from build123d import *

# Parameters (mm, degrees)
F0_R     = 8.575
F1_DEPTH = 26.5
F3_DEPTH = 26.5


with BuildPart() as f1:
    # F0 (on Top) → F1 (new body)
    with BuildSketch(Plane.XY):
        Circle(F0_R)
    extrude(amount=F1_DEPTH)

    # F2 (on face) → F3 (cut)
    with BuildSketch(Plane(origin=(0, 0, 0), x_dir=(1, 0, 0), z_dir=(0, 0, -1))):
        Polygon((4.9857674621, 0.3769917955), (2.3840555737, 1.6277629909), (2.6017118884, -1.2507711954), align=None)
        Polygon((2.819368203, -4.1293053818), (2.6017118884, -1.2507711954), (0.2176563146, -2.8785341864), align=None)
        Polygon((0.2176563146, -2.8785341864), (-2.3840555737, -1.6277629909), (-2.1663992591, -4.5062971773), align=None)
        Polygon((-2.3840555737, -1.6277629909), (-2.6017118884, 1.2507711954), (-4.9857674621, -0.3769917955), align=None)
        Polygon((2.3840555737, 1.6277629909), (-0.2176563146, 2.8785341864), (-2.6017118884, 1.2507711954), (-2.3840555737, -1.6277629909), (0.2176563146, -2.8785341864), (2.6017118884, -1.2507711954), align=None)
        Polygon((2.1663992591, 4.5062971773), (-0.2176563146, 2.8785341864), (2.3840555737, 1.6277629909), align=None)
        Polygon((-0.2176563146, 2.8785341864), (-2.819368203, 4.1293053818), (-2.6017118884, 1.2507711954), align=None)
    extrude(amount=-F3_DEPTH, mode=Mode.SUBTRACT)


solid = f1.part
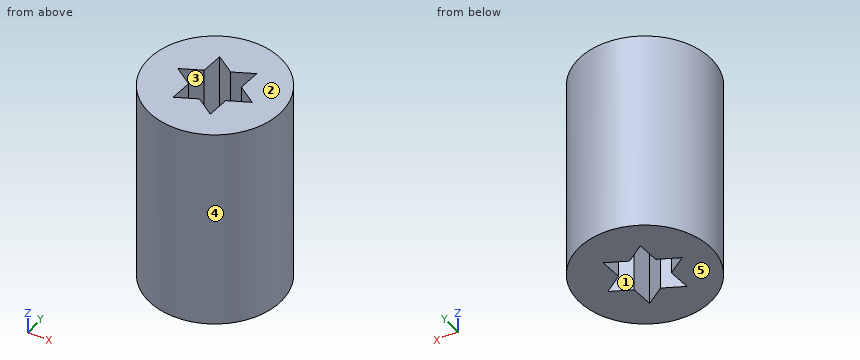
Design review of the part built by this model. Coordinates are the model's own, in mm. Face numbers are marked on the shaded views. A direction names the side the tool comes from. Round coordinates to 2 decimals unless told otherwise and drop trailing zeros. Write each loop counter-clockwise with the first axis right and the second up, starting at its lowest first coordinate (ties: lowest second). Pieces come first, ordered by that corner, then holes. Notation, with made-up numbers: (34.5, -9) - (82.5, -9) arc R14 ccw to (82.5, 7) - close; hole circle Ø6 at (60.5, 45). An arc over 180 degrees is marked (long way). Return JSON: item names as keys, results as strings. Group by question number.
Item 1: Machinability: for the marked faces 1 and 2, which of the approach directions +Z, -Z, +X, -X, +Y, -Y give a long, thin tool a straight path to every point of the face, cutting with its end or side? Answer none if there is none.
Item 2: The part is to be moulded in two halves that separate along Y. For the marked faces 3, 4 and 5, say which applies: pulls with the +Y half, pulls with the -Y half, needs draft (parallel to the pull), parting line crosses it, or undercut.
Item 3: We need section B-B on y = 0. Write out the cut boundary in (x, z) (3 decimals).
Item 4: We need section D-D on y = -5.75. Write out the cut boundary in (x, z), and give its area (3 significant figures).
Item 5: We need section A-A on z = 24.75. Write out the cut boundary in (x, y) (3 decimals), and give its area (3 significant figures).
Item 6: For probe 1 along X at (y, z) = (0.75, 2); probe 2 along X at (y, z) = (2, 13.75); probe 3 along Y at (x, z) = (3.5, 9), list the stretches that pass through material, from the lowest coordinate up. Write a range as [from, to].
Item 7: Insertion check: P1, Ø1, axis at x = 2.5, y = 0.5, coming from the -Z side; P2, Ø4, axis at y = -6.5, z = 13.5, coming from the -X side; P3, Ø2, axis at y = -3.5, z = 11, coming from the -X side; P4, Ø5, axis at y = -6, z = 8.5, coming from the -X side. Each pin has a flat end and moves straight along its axis. Give the tip position at first contact, or say it passes through.
Item 8: We need section C-C on y = 2. Write out the cut boundary in (x, z).
Model answer:
{
 "1": {"face 1": "+Z, -Z", "face 2": "+Z, +X, -X, +Y, -Y"},
 "2": {"face 3": "undercut", "face 4": "parting line crosses it", "face 5": "needs draft"},
 "3": {"outline": "(-8.575, 0) - (-4.434, 0) - (-4.434, 26.5) - (-8.575, 26.5) - close; (4.434, 0) - (8.575, 0) - (8.575, 26.5) - (4.434, 26.5) - close"},
 "4": {"outline": "(-6.36, 0) - (6.36, 0) - (6.36, 26.5) - (-6.36, 26.5) - close", "area": "337 mm²"},
 "5": {"outline": "circle Ø17.15 at (0, 0); hole (-4.986, 0.377) - (-2.602, -1.251) - (-2.819, -4.129) - (-0.218, -2.879) - (2.166, -4.506) - (2.384, -1.628) - (4.986, -0.377) - (2.602, 1.251) - (2.819, 4.129) - (0.218, 2.879) - (-2.166, 4.506) - (-2.384, 1.628) - close", "area": "188 mm²"},
 "6": {"probe 1": "x = [-8.54, -4.21], [3.34, 8.54]", "probe 2": "x = [-8.34, -2.36], [2.66, 8.34]", "probe 3": "y = [-7.83, -1.09], [0.64, 7.83]"},
 "7": {"P1": "passes through", "P2": "stops at x = -7.3", "P3": "stops at x = -8.2", "P4": "stops at x = -7.83"},
 "8": {"outline": "(-8.34, 0) - (-2.36, 0) - (-2.36, 26.5) - (-8.34, 26.5) - close; (2.66, 0) - (8.34, 0) - (8.34, 26.5) - (2.66, 26.5) - close"}
}
